Read the model definition and answer for the solid it produces. Units are mm, in the model's axes. A direction names the side the tool comes from. Coordinates: 2 decimals unless noted, no trailing zeros. Write each loop counter-clockwise with the first axis right and the second up, starting at its lowest first coordinate (ties: lowest second). Pieces come first, ordered by that corner, then holes. Notation, with made-up numbers: (43, 69) -> (66, 69) arc R23 cw to (66, 85) -> close; hole circle Ø8 at (-20.75, 17.5). An arc over 180 degrees is marked (long way). Use CSV: the item, a comma, the result in double quotes.
from build123d import *

# Parameters (mm, degrees)
F1_DEPTH = 50


with BuildPart() as f1:
    # F0 (on Front) → F1 (new body)
    with BuildSketch(Plane.XZ):
        with BuildLine():
            Line((0, 0), (0, 1))
            Line((0, 1), (-5, 1))
            Line((-5, 1), (-5, 0))
            Line((-5, 0), (-3, 0))
            Line((-3, 0), (-3, -2))
            ThreePointArc((-3, -2), (-3.414214, -3), (-3, -4))
            Line((-3, -4), (-2, -4))
            Line((-2, -4), (-2, 0))
            Line((-2, 0), (0, 0))
        make_face()
    extrude(amount=F1_DEPTH)

    # F2: F1 across plane


with BuildPart() as f1_1:
    add(f1.part)
    add(f1.part.mirror(Plane.YZ))


solid = f1_1.part
1. A cutting plane is placed at C-C (x = -1). Give the vertices of the cut face in (y, z), and give its area (3 significant figures).
Solutions:
outline,"(-50, 0) -> (0, 0) -> (0, 1) -> (-50, 1) -> close"
area,"50.0 mm^2"
2. A tool of negligible diameter and unlimited length cuts with its end or side. For faces 4 (the flat face through (3, -25, -1)), 5 (the flat face through (2, -25, -2)), 6 (the flat face through (-3, -25, -1)), from which of +Z, -Z, +X, -X, +Y, -Y can it reach the whole face along a straight path? Write none if from no direction.
Solutions:
face 4,"+X, +Y, -Y"
face 5,"-Z, +Y, -Y"
face 6,"-X, +Y, -Y"
3. Each of these flat-tipped pins is pushed along its axis until it touches: pin 1 Ø1 at (x, z) = (4, -2.5) entering from -Y; pin 2 Ø2 at (y, z) = (-14, -1.5) entering from -X; pin 3 Ø0.6 at (x, y) = (3.5, -27) entering from -Z; pin 4 Ø3 at (y, z) = (-13, -2) entering from -X. Where does it stop, or does it pass through?
Solutions:
pin 1,"passes through"
pin 2,"stops at x = -3.32"
pin 3,"stops at z = -3.75"
pin 4,"stops at x = -3.41"
4. Find the intervals of material crossed by line 1 along X through (y, z) = (-31, -1.85); line 2 along X through (y, z) = (-6, -2.9); line 3 along Z through (x, y) = (1.25, -19.5), in increasing order.
Solutions:
line 1,"x = -3 to -2, 2 to 3"
line 2,"x = -3.41 to -2, 2 to 3.41"
line 3,"z = 0 to 1"
5. A cutting plane is placed at B-B (y = -10.5). Give the vertices of the cut face in (x, z), and give its area (3 significant figures).
Solutions:
outline,"(-5, 0) -> (-3, 0) -> (-3, -2) arc R1.41 ccw to (-3, -4) -> (-2, -4) -> (-2, 0) -> (2, 0) -> (2, -4) -> (3, -4) arc R1.41 ccw to (3, -2) -> (3, 0) -> (5, 0) -> (5, 1) -> (-5, 1) -> close"
area,"19.1 mm^2"
6. A cutting plane is placed at A-A (z = -1.35). Give the vertices of the cut face in (x, y).
Solutions:
outline,"(-3, -50) -> (-2, -50) -> (-2, 0) -> (-3, 0) -> close; (2, -50) -> (3, -50) -> (3, 0) -> (2, 0) -> close"
7. For a pull along X with two mould halves and no side action, classify faces 1 (the flat face through (0, -25, 0)), 2 (the flat face through (0.1, -50, 0.2)), 3 (the flat face through (5, -24.6, 0.5)) as pulls with the +X half, pulls with the -X half, needs draft (parallel to the pull), parting line crosses it, or undercut.
Solutions:
face 1,"undercut"
face 2,"needs draft"
face 3,"pulls with the +X half"
